Solid Edge part; units mm, degrees
sketch "Sketch1" plane through (0, 0, 0) normal (0, 0, 1) x (1, 0, 0)
  circle A0 centre (0, 0) radius 4.5
  circle A1 centre (0, 0) radius 2.5
extrude "Protrusion1" add sketch "Sketch1" along normal mid plane 10
fillet "Round_1" radius 0.5 2 edges at (-2.5, 0, -5) (-2.5, 0, 5)
fillet "Round_2" radius 0.5 2 edges at (-4.5, 0, -5) (-4.5, 0, 5)
properties material "Acrylic, high impact grade"
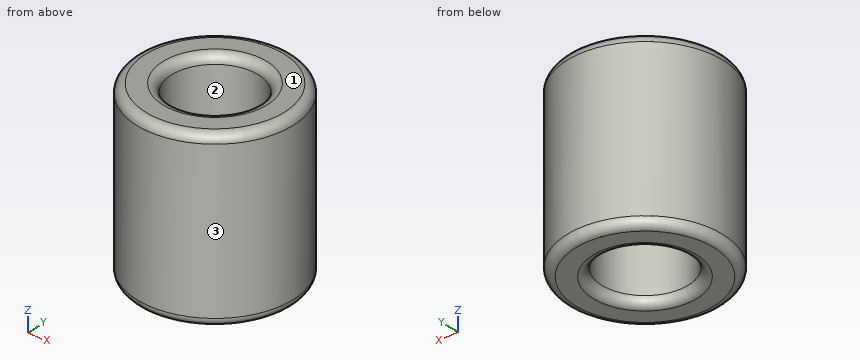
Verification items for the finished model (mm, model axes). Face numbers are marked on the shaded views. Round coordinates to 2 decimals unless told otherwise and drop trailing zeros. Loops run counter-clockwise (first coordinate to the right, second up) from the corner with the lowest first, then second, coordinate; pieces in that order, holes last. Notation, with made-up numbers: (0, -29) - (33, -29) arc R29 ccw to (33, 4) - close; hole circle Ø4 at (89, 80). An arc over 180 degrees is marked (long way). Use one line per item in the form item = value.
1. Scan lines: probe 1 along Y at (x, z) = (0, -2); probe 2 along X at (y, z) = (1.75, -2.5); probe 3 along X at (y, z) = (-0.75, -0.5). Record each from-to range of solid material in increasing order.
A:
probe_1 = -4.5 to -2.5, 2.5 to 4.5
probe_2 = -4.15 to -1.79, 1.79 to 4.15
probe_3 = -4.44 to -2.38, 2.38 to 4.44
2. Section check A-A on y = 0. Record the cut outline in (x, z).
A:
outline = (-4.5, -4.5) arc R0.5 ccw to (-4, -5) - (-3, -5) arc R0.5 ccw to (-2.5, -4.5) - (-2.5, 4.5) arc R0.5 ccw to (-3, 5) - (-4, 5) arc R0.5 ccw to (-4.5, 4.5) - close; (2.5, -4.5) arc R0.5 ccw to (3, -5) - (4, -5) arc R0.5 ccw to (4.5, -4.5) - (4.5, 4.5) arc R0.5 ccw to (4, 5) - (3, 5) arc R0.5 ccw to (2.5, 4.5) - close
3. Draft check along Y on the marked faces 1, 2 and 3. Enter one of: pulls with the +Y half, pulls with the -Y half, needs draft (parallel to the pull), parting line crosses it, or undercut.
A:
face_1 = needs draft
face_2 = undercut
face_3 = parting line crosses it
4. Section check C-C on z = -3. Record the cut outline in (x, y).
A:
outline = circle Ø9 at (0, 0); hole circle Ø5 at (0, 0)
5. Gauge pin test, flat ends, axial feed: pin 1 Ø1.5 at (y, z) = (-3.5, 3) entering from +X; pin 2 Ø1.5 at (y, z) = (-2.5, 1) entering from -X. Record the tip position at first contact, or that the pin passes through.
A:
pin_1 = 3.56
pin_2 = -4.15
